```python
from build123d import *

# Parameters (mm, degrees)
SKETCH1_R           = 3.5
SKETCH1_R_2         = 6
BOSS_EXTRUDE1_DEPTH = 3


with BuildPart() as part:
    # Sketch1 → Boss-Extrude1 (new body)
    with BuildSketch(Plane.XY):
        with BuildLine():
            Line((0, 20), (0, 0))
            Line((0, 0), (145, 0))
            Line((145, 0), (145, 5))
            Line((145, 5), (115.5, 5))
            ThreePointArc((115.5, 5), (112, 8.5), (115.5, 12))
            Line((115.5, 12), (145, 12))
            Line((145, 12), (145, 20))
            Line((145, 20), (0, 20))
        make_face()
        with Locations((30, 10)):
            Circle(SKETCH1_R, mode=Mode.SUBTRACT)
        with Locations((67, 10)):
            Circle(SKETCH1_R_2, mode=Mode.SUBTRACT)
        with Locations((95, 10)):
            Circle(SKETCH1_R_2, mode=Mode.SUBTRACT)
    extrude(amount=BOSS_EXTRUDE1_DEPTH)


solid = part.part
```
Model file for the job. Use its own axes, mm. A direction names the side the tool comes from. Round coordinates to 2 decimals unless told otherwise and drop trailing zeros. Order: outer loops, then holes, each group sorted by start corner. A loop starts at its lowest first (then second) coordinate and runs counter-clockwise, first axis right, second up. Notation, with made-up numbers: M 65,1 L 103,1 A16 ccw 103,29 Z; hole C -16,44 d7. An arc over 180 degrees is marked long. Use CSV: the item, a comma, the result in double quotes.
Item 1: Saw through at A-A (x = 30). List the corners of the cut face in (y, z).
Worked answers:
outline,"M 0,0 L 6.5,0 L 6.5,3 L 0,3 Z; M 13.5,0 L 20,0 L 20,3 L 13.5,3 Z"
Item 2: Saw through at D-D (x = 92). List the corners of the cut face in (y, z), plus the area to 3 significant figures.
Worked answers:
outline,"M 0,0 L 4.8,0 L 4.8,3 L 0,3 Z; M 15.2,0 L 20,0 L 20,3 L 15.2,3 Z"
area,"28.8 mm²"
Item 3: Which spindle directions (+Z, -Z, +X, -X, +Y, -Y) get a long thin tool onto all of the face, cutting with end or side? Do faces 1 (the face through (71, 15, 0)), 2 (the face through (130, 5, 1)). Say none if no direction does.
Worked answers:
face 1,"-Z, +X, -X, +Y, -Y"
face 2,"+Z, -Z, +X"
Item 4: Probe probe 1 along X at (y, z) = (7.5, 1.3); probe 2 along X at (y, z) = (15.25, 0.4); probe 3 along X at (y, z) = (8.5, 2.15). List the from-to ranges inside material, lowest first.
Worked answers:
probe 1,"0 to 27.55, 32.45 to 61.55, 72.45 to 89.55, 100.45 to 112.15"
probe 2,"0 to 64.1, 69.9 to 92.1, 97.9 to 145"
probe 3,"0 to 26.84, 33.16 to 61.19, 72.81 to 89.19, 100.81 to 112"
Item 5: Saw through at B-B (z = 1.3). List the corners of the cut face in (x, y), plus the area to 3 significant figures.
Worked answers:
outline,"M 0,0 L 145,0 L 145,5 L 115.5,5 A3.5 cw 115.5,12 L 145,12 L 145,20 L 0,20 Z; hole C 30,10 d7; hole C 67,10 d12; hole C 95,10 d12"
area,"2,410 mm²"
Item 6: Saw through at C-C (y = 7.75). List the corners of the cut face in (x, z).
Worked answers:
outline,"M 0,0 L 27.32,0 L 27.32,3 L 0,3 Z; M 32.68,0 L 61.44,0 L 61.44,3 L 32.68,3 Z; M 72.56,0 L 89.44,0 L 89.44,3 L 72.56,3 Z; M 100.56,0 L 112.08,0 L 112.08,3 L 100.56,3 Z"
Item 7: Pull direction X, two halves, no side cores. Call faces 3 (the face through (130, 12, 1)), 4 (the face through (145, 2, 1)), 5 (the face through (0, 10, 1)), 6 (the face through (89, 10, 1)): released by +X, released by -X, zero draft, split by the parting line, or undercut.
Worked answers:
face 3,"zero draft"
face 4,"released by +X"
face 5,"released by -X"
face 6,"undercut"
